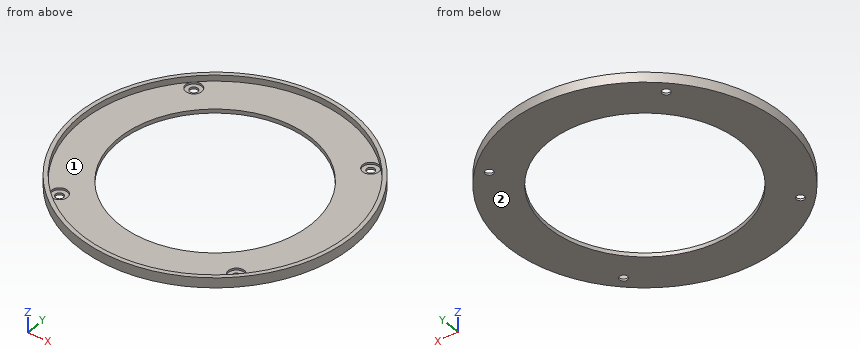
```python
from build123d import *

# Parameters (mm, degrees)
F0_R     = 54.477198
F0_R_2   = 1.5875
F0_R_3   = 38.1
F1_DEPTH = 1.5875
F2_R     = 54.477198
F2_R_2   = 52.889698
F3_DEPTH = 2.38125
F4_R     = 3.175
F5_DEPTH = 0.79375


with BuildPart() as f1:
    # F0 (on Top) → F1 (new body)
    with BuildSketch(Plane.XY):
        Circle(F0_R)
        with Locations((-35.1536, -35.1536)):
            Circle(F0_R_2, mode=Mode.SUBTRACT)
        with Locations((35.1536, -35.1536)):
            Circle(F0_R_2, mode=Mode.SUBTRACT)
        with Locations((-35.1536, 35.1536)):
            Circle(F0_R_2, mode=Mode.SUBTRACT)
        Circle(F0_R_3, mode=Mode.SUBTRACT)
        with Locations((35.1536, 35.1536)):
            Circle(F0_R_2, mode=Mode.SUBTRACT)
    extrude(amount=F1_DEPTH)

    # F2 (on face) → F3 (join)
    with BuildSketch(Plane.XY.offset(1.5875)):
        Circle(F2_R)
        Circle(F2_R_2, mode=Mode.SUBTRACT)
    extrude(amount=F3_DEPTH)

    # F4 (on face) → F5 (cut)
    with BuildSketch(Plane.XY.offset(1.5875)):
        with Locations((-35.1536, 35.1536)):
            Circle(F4_R)
        with Locations((35.1536, 35.1536)):
            Circle(F4_R)
        with Locations((35.1536, -35.1536)):
            Circle(F4_R)
        with Locations((-35.1536, -35.1536)):
            Circle(F4_R)
    extrude(amount=-F5_DEPTH, mode=Mode.SUBTRACT)


solid = f1.part
```
Here's how the part is built. I have some questions about the finished solid (model axes, mm). Face numbers are marked on the shaded views. Round coordinates to 2 decimals unless told otherwise and drop trailing zeros. Order: outer loops, then holes, each group sorted by start corner. A loop starts at its lowest first (then second) coordinate and runs counter-clockwise, first axis right, second up. Notation, with made-up numbers: M -6.75,-12.75 L 35.25,-12.75 A28 cw 35.25,18.25 Z; hole C -37,23 d7. An arc over 180 degrees is marked long. Use CSV: the item, a comma, the result in double quotes.
1) I'm going to push flat-ended pins straight in: P1, Ø1.9, axis at x = 35.15, y = -35.15, coming from the +Z side; P2, Ø1.5, axis at x = -36.5, z = 3, coming from the +Y side; P3, Ø4, axis at x = -35.15, y = 35.15, coming from the +Z side; P4, Ø3, axis at x = -34, y = 36.5, coming from the +Z side. Where does each tip first touch, or does it pass through?
Taken from the geometry:
P1,"through"
P2,"y = 41.11"
P3,"z = 0.79"
P4,"z = 1.59"
2) If we mould it in two halves opening along Z, with no side actions, what happens to the marked faces 1 and 2? For each: pulls with the +Z half, pulls with the -Z half, needs draft (parallel to the pull), parting line crosses it, or undercut.
Taken from the geometry:
face 1,"pulls with the +Z half"
face 2,"pulls with the -Z half"
3) I want a section at A-A (x = 0). List the corners of the cut face in (y, z) for me, then the cut area to 3 significant figures.
Taken from the geometry:
outline,"M -54.48,0 L -38.1,0 L -38.1,1.59 L -52.89,1.59 L -52.89,3.97 L -54.48,3.97 Z; M 38.1,0 L 54.48,0 L 54.48,3.97 L 52.89,3.97 L 52.89,1.59 L 38.1,1.59 Z"
area,"59.6 mm^2"
4) I want a section at C-C (z = 2.8). List the corners of the cut face in (x, y) for me.
Taken from the geometry:
outline,"C 0,0 d108.95; hole C 0,0 d105.78"
5) I need wall thicknesses on line 1 along X through (y, z) = (35, 0.7); line 2 along Z through (x, y) = (-47, -15.5); line 3 along Y through (x, z) = (-15.5, 2.1). Which ranges of each line are inside material? Lowest first, please. Write a range as [from, to].
Taken from the geometry:
line 1,"[-41.75, -36.73], [-33.57, -15.05], [15.05, 33.57], [36.73, 41.75]"
line 2,"[0, 1.59]"
line 3,"[-52.23, -50.57], [50.57, 52.23]"
